Part model, mm, in its own coordinate system. Face numbers are marked on the shaded views. A direction names the side the tool comes from. Give positions to 0.01 mm unless a question says otherwise; leave off trailing zeros. Order: outer loops, then holes, each group sorted by start corner. A loop starts at its lowest first (then second) coordinate and runs counter-clockwise, first axis right, second up. Notation, with made-up numbers: (35, -3) - (45, -3) arc R15 cw to (45, 8) - close; hole circle Ø11 at (-12.75, 50). An arc over 180 degrees is marked (long way). Use one line per item in the form item = value. Start each with the question number.
1. Drill centre lines: line 1 (X direction, y = 1.6, z = -60.96); line 2 (Z direction, x = 35, y = 2); line 3 (Z direction, x = 86, y = 29). Where is each one in solid material? Low to high.
2. Pin check, flat tips, straight feed: P1, Ø5, axis at y = 9, z = -40, coming from the -X side; P2, Ø8.5, axis at x = 84.5, y = 24.5, coming from the -Z side; P3, Ø2.5, axis at y = 27, z = -65, coming from the +X side; P4, Ø11.5, axis at x = 81, y = 17, coming from the +Z side. Stop position of each tip, or through.
3. Tool access for the marked faces 3, 4, 5 and 6: list every direction of +Z, -Z, +X, -X, +Y, -Y with a clear straight run to the whole face (end or side of a thin tool).
4. Band-saw the part on D-D, the plane x = 86.36. List the corners of the cut face in (y, z).
5. Band-saw the part on A-A, the plane z = -40.5. List the corners of the cut face in (x, y), plus the area to 3 significant figures.
6. Pull direction X, two halves, no side cores. Call the marked faces 1 and 2: +X half, -X half, draft (parallel to the pull), parting line (faces both ways), or undercut.
7. Band-saw the part on C-C, the plane x = 20.32. List the corners of the cut face in (y, z), plus the area to 3 significant figures.
8. Band-saw the part on B-B, the plane y = 14.5. List the corners of the cut face in (x, z), plus the area to 3 significant figures.
from build123d import *

# Parameters (mm, degrees)
SKETCH1_W           = 93.98
SKETCH1_H           = 71.12
BOSS_EXTRUDE1_DEPTH = 5.08
FILLET4_R           = 5.08
CUT_EXTRUDE5_REACH  = 119.967
SKETCH7_R           = 3.429
SKETCH7_W           = 13.208
SKETCH7_H           = 19.558
CUT_EXTRUDE7_DEPTH  = 2.54
CUT_EXTRUDE8_REACH  = 119.967
SKETCH8_R           = 3.81
SKETCH2_W           = 7.874
SKETCH2_H           = 7.874
BOSS_EXTRUDE3_DEPTH = 30.48
SKETCH10_R          = 1.27
CUT_EXTRUDE9_DEPTH  = 12.7
FILLET5_R           = 2.286
CHAMFER4_SIZE       = 5.08
SKETCH11_W          = 103.535361548
SKETCH11_H          = 78.086950251
CUT_EXTRUDE10_DEPTH = 2.54


with BuildPart() as part:
    # Sketch1 → Boss-Extrude1 (new body)
    with BuildSketch(Plane(origin=(0, 0, 0), x_dir=(1, 0, 0), z_dir=(0, 1, 0))):
        with Locations((46.99, 35.56)):
            Rectangle(SKETCH1_W, SKETCH1_H)
    extrude(amount=BOSS_EXTRUDE1_DEPTH)

    # Fillet4
    fillet4_edges = [part.edges().sort_by_distance(p)[0] for p in [
        (0, 2.54, -71.12),
        (93.98, 2.54, -71.12),
        (93.98, 2.54, 0),
        (0, 2.54, 0),
    ]]
    fillet(fillet4_edges, radius=FILLET4_R)

    # Sketch7 → Cut-Extrude5 (cut, up to next)
    with BuildSketch(Plane(origin=(0, 5.08, 0), x_dir=(1, 0, 0), z_dir=(0, 1, 0)), mode=Mode.PRIVATE) as cut_extrude5_sk1:
        with Locations(Location((55.372, 45.339, 0), (0, 0, 270))):
            Circle(SKETCH7_R)
    cut_extrude5_tool1 = extrude(cut_extrude5_sk1.sketch, amount=-CUT_EXTRUDE5_REACH, mode=Mode.PRIVATE) & part.part
    # Sketch7 → Cut-Extrude5 (cut, up to next)
    with BuildSketch(Plane(origin=(0, 5.08, 0), x_dir=(1, 0, 0), z_dir=(0, 1, 0)), mode=Mode.PRIVATE) as cut_extrude5_sk2:
        with Locations(Location((55.372, 25.781, 0), (0, 0, 270))):
            Circle(SKETCH7_R)
    cut_extrude5_tool2 = extrude(cut_extrude5_sk2.sketch, amount=-CUT_EXTRUDE5_REACH, mode=Mode.PRIVATE) & part.part
    # Sketch7 → Cut-Extrude5 (cut, up to next)
    with BuildSketch(Plane(origin=(0, 5.08, 0), x_dir=(1, 0, 0), z_dir=(0, 1, 0)), mode=Mode.PRIVATE) as cut_extrude5_sk3:
        with Locations((72.136, 35.56)):
            Rectangle(SKETCH7_W, SKETCH7_H)
    cut_extrude5_tool3 = extrude(cut_extrude5_sk3.sketch, amount=-CUT_EXTRUDE5_REACH, mode=Mode.PRIVATE) & part.part
    add(cut_extrude5_tool1.solids().sort_by_distance((55.372, 5.08, -45.339))[0], mode=Mode.SUBTRACT)
    add(cut_extrude5_tool2.solids().sort_by_distance((55.372, 5.08, -25.781))[0], mode=Mode.SUBTRACT)
    add(cut_extrude5_tool3.solids().sort_by_distance((72.136, 5.08, -35.56))[0], mode=Mode.SUBTRACT)

    # Sketch9 → Cut-Extrude7 (cut)
    with BuildSketch(Plane(origin=(0, 5.08, 0), x_dir=(1, 0, 0), z_dir=(0, 1, 0))):
        with BuildLine():
            Line((49.022, 45.339), (49.022, 25.781))
            ThreePointArc((49.022, 25.781), (50.881871939, 21.290871939), (55.372, 19.431))
            Line((55.372, 19.431), (65.532, 19.431))
            Line((65.532, 19.431), (78.74, 19.431))
            Line((78.74, 19.431), (78.74, 51.689))
            Line((78.74, 51.689), (65.532, 51.689))
            Line((65.532, 51.689), (55.372, 51.689))
            ThreePointArc((55.372, 51.689), (50.881871939, 49.829128061), (49.022, 45.339))
        make_face()
    extrude(amount=-CUT_EXTRUDE7_DEPTH, mode=Mode.SUBTRACT)

    # Sketch8 → Cut-Extrude8 (cut, up to next)
    with BuildSketch(Plane(origin=(0, 5.08, 0), x_dir=(1, 0, 0), z_dir=(0, 1, 0)), mode=Mode.PRIVATE) as cut_extrude8_sk1:
        with Locations(Location((20.32, 10.16, 0), (0, 0, 270))):
            Circle(SKETCH8_R)
    cut_extrude8_tool1 = extrude(cut_extrude8_sk1.sketch, amount=-CUT_EXTRUDE8_REACH, mode=Mode.PRIVATE) & part.part
    # Sketch8 → Cut-Extrude8 (cut, up to next)
    with BuildSketch(Plane(origin=(0, 5.08, 0), x_dir=(1, 0, 0), z_dir=(0, 1, 0)), mode=Mode.PRIVATE) as cut_extrude8_sk2:
        with Locations(Location((35.56, 10.16, 0), (0, 0, 270))):
            Circle(SKETCH8_R)
    cut_extrude8_tool2 = extrude(cut_extrude8_sk2.sketch, amount=-CUT_EXTRUDE8_REACH, mode=Mode.PRIVATE) & part.part
    # Sketch8 → Cut-Extrude8 (cut, up to next)
    with BuildSketch(Plane(origin=(0, 5.08, 0), x_dir=(1, 0, 0), z_dir=(0, 1, 0)), mode=Mode.PRIVATE) as cut_extrude8_sk3:
        with Locations(Location((35.56, 60.96, 0), (0, 0, 90))):
            Circle(SKETCH8_R)
    cut_extrude8_tool3 = extrude(cut_extrude8_sk3.sketch, amount=-CUT_EXTRUDE8_REACH, mode=Mode.PRIVATE) & part.part
    # Sketch8 → Cut-Extrude8 (cut, up to next)
    with BuildSketch(Plane(origin=(0, 5.08, 0), x_dir=(1, 0, 0), z_dir=(0, 1, 0)), mode=Mode.PRIVATE) as cut_extrude8_sk4:
        with Locations(Location((20.32, 60.96, 0), (0, 0, 90))):
            Circle(SKETCH8_R)
    cut_extrude8_tool4 = extrude(cut_extrude8_sk4.sketch, amount=-CUT_EXTRUDE8_REACH, mode=Mode.PRIVATE) & part.part
    add(cut_extrude8_tool1.solids().sort_by_distance((20.32, 5.08, -10.16))[0], mode=Mode.SUBTRACT)
    add(cut_extrude8_tool2.solids().sort_by_distance((35.56, 5.08, -10.16))[0], mode=Mode.SUBTRACT)
    add(cut_extrude8_tool3.solids().sort_by_distance((35.56, 5.08, -60.96))[0], mode=Mode.SUBTRACT)
    add(cut_extrude8_tool4.solids().sort_by_distance((20.32, 5.08, -60.96))[0], mode=Mode.SUBTRACT)

    # Sketch2 → Boss-Extrude3 (add)
    with BuildSketch(Plane(origin=(0, 5.08, 0), x_dir=(1, 0, 0), z_dir=(0, 1, 0))):
        with Locations((6.731, 64.389)):
            Rectangle(SKETCH2_W, SKETCH2_H)
        with Locations((87.249, 64.389)):
            Rectangle(SKETCH2_W, SKETCH2_H)
        with Locations((87.249, 6.731)):
            Rectangle(SKETCH2_W, SKETCH2_H)
        with Locations((6.731, 6.731)):
            Rectangle(SKETCH2_W, SKETCH2_H)
    extrude(amount=BOSS_EXTRUDE3_DEPTH)

    # Sketch10 → Cut-Extrude9 (cut)
    with BuildSketch(Plane(origin=(0, 35.56, 0), x_dir=(1, 0, 0), z_dir=(0, 1, 0))):
        with Locations(Location((7.62, 63.5, 0), (0, 0, 270))):
            Circle(SKETCH10_R)
        with Locations(Location((86.36, 63.5, 0), (0, 0, 90))):
            Circle(SKETCH10_R)
        with Locations(Location((86.36, 7.62, 0), (0, 0, 270))):
            Circle(SKETCH10_R)
        with Locations(Location((7.62, 7.62, 0), (0, 0, 90))):
            Circle(SKETCH10_R)
    extrude(amount=-CUT_EXTRUDE9_DEPTH, mode=Mode.SUBTRACT)

    # Fillet5
    fillet5_edges = [part.edges().sort_by_distance(p)[0] for p in [
        (2.794, 20.32, -68.326),
        (91.186, 20.32, -68.326),
        (91.186, 20.32, -2.794),
        (2.794, 20.32, -2.794),
    ]]
    fillet(fillet5_edges, radius=FILLET5_R)

    # Chamfer4
    chamfer4_edges = [part.edges().sort_by_distance(p)[0] for p in [
        (6.731, 5.08, -60.452),
        (10.668, 5.08, -64.389),
        (83.312, 5.08, -64.389),
        (87.249, 5.08, -60.452),
        (87.249, 5.08, -10.668),
        (83.312, 5.08, -6.731),
        (10.668, 5.08, -6.731),
        (6.731, 5.08, -10.668),
    ]]
    chamfer(chamfer4_edges, length=CHAMFER4_SIZE)

    # Sketch11 → Cut-Extrude10 (cut)
    with BuildSketch(Plane(origin=(0, 35.56, 0), x_dir=(1, 0, 0), z_dir=(0, 1, 0))):
        with Locations((47.570572121, 35.36647596)):
            Rectangle(SKETCH11_W, SKETCH11_H)
    extrude(amount=-CUT_EXTRUDE10_DEPTH, mode=Mode.SUBTRACT)


solid = part.part
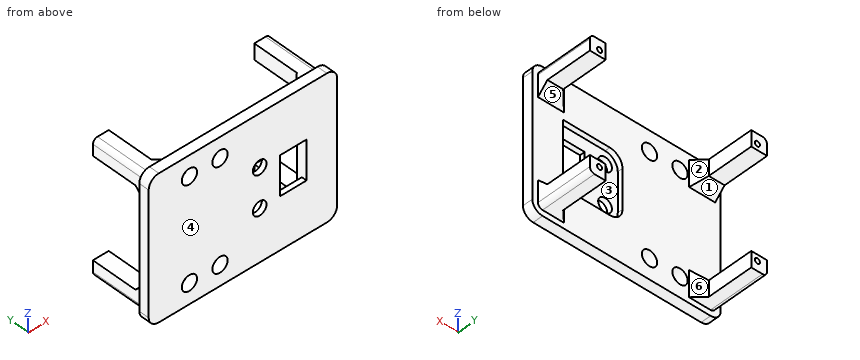
From the geometry:
q1.line_1 = 0 to 16.51, 24.13 to 31.75, 39.37 to 93.98
q1.line_2 = -71.12 to -64.73, -57.19 to -13.93, -6.39 to 0
q1.line_3 = -68.33 to -64.72, -62.28 to -60.45, -10.67 to -8.84, -6.4 to -2.79
q2.P1 = through
q2.P2 = -68.33
q2.P3 = 91.19
q2.P4 = -2.79
q3.face_3 = +Y
q3.face_4 = +Z, -Z, +X, -X, -Y
q3.face_5 = +X, -X, +Y
q3.face_6 = +Z, -Z, +Y
q4.outline = (0, -71.12) - (5.08, -71.12) - (5.08, -68.33) - (33.02, -68.33) - (33.02, -64.77) - (22.86, -64.77) - (22.86, -62.23) - (33.02, -62.23) - (33.02, -60.45) - (10.16, -60.45) - (5.08, -55.37) - (5.08, -15.75) - (10.16, -10.67) - (33.02, -10.67) - (33.02, -8.89) - (22.86, -8.89) - (22.86, -6.35) - (33.02, -6.35) - (33.02, -2.79) - (5.08, -2.79) - (5.08, 0) - (0, 0) - close
q5.outline = (0, 0) - (65.53, 0) - (65.53, 2.54) - (49.02, 2.54) - (49.02, 5.08) - (0, 5.08) - close; (78.74, 0) - (93.98, 0) - (93.98, 5.08) - (78.74, 5.08) - close
q5.area = 368 mm²
q6.face_1 = draft
q6.face_2 = undercut
q7.outline = (0, -71.12) - (5.08, -71.12) - (5.08, -64.77) - (0, -64.77) - close; (0, -57.15) - (5.08, -57.15) - (5.08, -13.97) - (0, -13.97) - close; (0, -6.35) - (5.08, -6.35) - (5.08, 0) - (0, 0) - close
q7.area = 284 mm²
q8.outline = (2.79, -66.04) arc R2.29 ccw to (5.08, -68.33) - (10.67, -68.33) - (10.67, -60.45) - (2.79, -60.45) - close; (2.79, -10.67) - (10.67, -10.67) - (10.67, -2.79) - (5.08, -2.79) arc R2.29 ccw to (2.79, -5.08) - close; (83.31, -68.33) - (88.9, -68.33) arc R2.29 ccw to (91.19, -66.04) - (91.19, -60.45) - (83.31, -60.45) - close; (83.31, -10.67) - (91.19, -10.67) - (91.19, -5.08) arc R2.29 ccw to (88.9, -2.79) - (83.31, -2.79) - close
q8.area = 244 mm²
